```python
from build123d import *

# Parameters (mm, degrees)
D24_5_5_D6_5_2_R                = 12
D24_5_5_D6_5_2_R_2              = 3.25
D24_5_5_D6_5_DEPTH              = 5.5
EXTRUDE_START                   = 5.5
SKETCH_D9_8_1_5_R               = 4.9
SKETCH_D9_8_1_5_R_2             = 3.25
EXTRUDE_D9_8_1_5_DEPTH          = 1.5
F_4XD3_4_D5_8_PCD16_D           = 3.4
F_4XD3_4_D5_8_PCD16_CBORE_D     = 5.8
F_4XD3_4_D5_8_PCD16_CBORE_DEPTH = 3.8
SKETCH_1093_R                   = 10.05
CUT_EXTRUDE_D20_1_0_6_DEPTH     = 0.6
F_4XM2X0_4_PCD14_D              = 1.6


with BuildPart() as part:
    # D24__5.5__D6.5 2 → D24__5.5__D6.5 (new body)
    with BuildSketch(Plane.XY):
        Circle(D24_5_5_D6_5_2_R)
        Circle(D24_5_5_D6_5_2_R_2, mode=Mode.SUBTRACT)
    extrude(amount=D24_5_5_D6_5_DEPTH)

    # 轴承内孔定位台_D9.8_高1.5_截面 → 轴承内孔定位台_D9.8_高1.5 (add)
    with BuildSketch(Plane.XY.offset(EXTRUDE_START)):
        Circle(SKETCH_D9_8_1_5_R)
        Circle(SKETCH_D9_8_1_5_R_2, mode=Mode.SUBTRACT)
    extrude(amount=EXTRUDE_D9_8_1_5_DEPTH)

    # 轴承内圈_4xD3.4通孔_D5.8沉孔_PCD16 (through all)
    with Locations(Plane(origin=(5.656854249, -5.656854249, 0), x_dir=(-1, 0, 0), z_dir=(0, 0, -1))):
        with Locations((0, 0), (11.313708498, 0), (11.313708498, 11.313708498), (0, 11.313708498)):
            CounterBoreHole(F_4XD3_4_D5_8_PCD16_D / 2, F_4XD3_4_D5_8_PCD16_CBORE_D / 2, F_4XD3_4_D5_8_PCD16_CBORE_DEPTH)

    # Sketch 1093 → 原舵盘定位槽_D20.1_深0.6 (cut)
    with BuildSketch(Plane.XY):
        Circle(SKETCH_1093_R)
    extrude(amount=CUT_EXTRUDE_D20_1_0_6_DEPTH, mode=Mode.SUBTRACT)

    # 原舵盘_4xM2x0.4通螺纹_PCD14 (through all)
    with Locations(Plane(origin=(0, -7, 0.6), x_dir=(-1, 0, 0), z_dir=(0, 0, -1))):
        with Locations((0, 0), (7, 7), (0, 14), (-7, 7)):
            Hole(F_4XM2X0_4_PCD14_D / 2)


solid = part.part
```
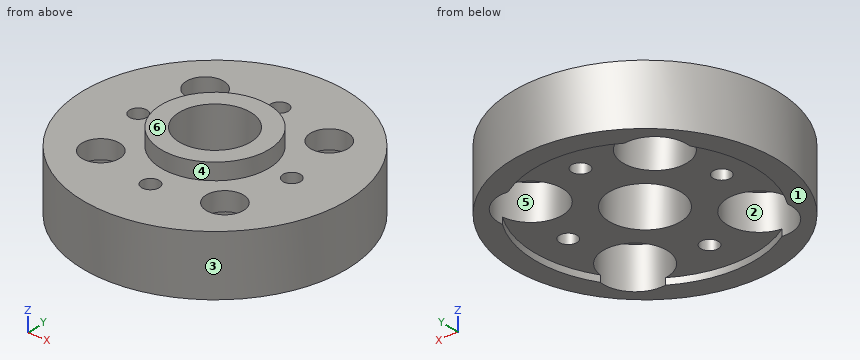
The model under review builds one solid part; all positions refer to its coordinate system, in mm. Face numbers are marked on the shaded views. A direction names the side the tool comes from. Coordinates: 2 decimals unless noted, no trailing zeros. Order: outer loops, then holes, each group sorted by start corner. A loop starts at its lowest first (then second) coordinate and runs counter-clockwise, first axis right, second up. Notation, with made-up numbers: (54, 52) -> (104, 52) arc R26 ccw to (104, 74) -> close; hole circle Ø5 at (83.25, -34). An arc over 180 degrees is marked (long way). Answer in a Markdown table with one row per item. Add a question column.
Item 1: Machinability: for the marked faces 4, 5 and 6, which of the approach directions +Z, -Z, +X, -X, +Y, -Y give a long, thin tool a straight path to every point of the face, cutting with its end or side? Answer none if there is none.
Item 2: We need section B-B on y = -4.5. Write out the cut boundary in (x, z), plus the area to 3 significant figures.
Item 3: To check wall thickness, follow probe 1 along Y at (x, z) = (4, 2.5); probe 2 along X at (y, z) = (-4.5, 5.25); probe 3 along X at (y, z) = (-5.5, 4). State the ranges of each line that lie inside material, in increasing order.
Item 4: Clearance check with flat-ended pins moving along their axes: pin 1 (5.5 mm diameter, centred on x = -5.66, y = 5.66, fed in from +Z); pin 2 (2 mm diameter, centred on y = 5, z = 4.5, fed in from -X); pin 3 (6.5 mm diameter, centred on x = -6.5, y = 6.5, fed in from -Z); pin 4 (2 mm diameter, centred on x = -7, y = 0, fed in from -Z). State where each tip first meets the part, or that it passes through.
Item 5: Mouldability with a two-part tool opening along X and no side actions: class the marked faces 1, 2 and 3 as +X half, -X half, draft (parallel to the pull), parting line (faces both ways), or undercut.
Item 6: We need section A-A on x = 0. Write out the cut boundary in (y, z), plus the area to 3 significant figures.
Item 7: We need section D-D on z = 6.5. Write out the cut boundary in (x, y).
Final values:
| question | item | result |
|---|---|---|
| 1 | face 4 | +Z |
| 1 | face 5 | -Z |
| 1 | face 6 | +Z, +X, -X, +Y, -Y |
| 2 | outline | (-11.12, 0) -> (-8.99, 0) -> (-8.99, 0.6) -> (-8.32, 0.6) -> (-8.32, 3.8) -> (-6.9, 3.8) -> (-6.9, 5.5) -> (-11.12, 5.5) -> close; (-4.41, 3.8) -> (-3, 3.8) -> (-3, 0.6) -> (3, 0.6) -> (3, 3.8) -> (4.41, 3.8) -> (4.41, 5.5) -> (1.94, 5.5) -> (1.94, 7) -> (-1.94, 7) -> (-1.94, 5.5) -> (-4.41, 5.5) -> close; (6.9, 3.8) -> (8.32, 3.8) -> (8.32, 0.6) -> (8.99, 0.6) -> (8.99, 0) -> (11.12, 0) -> (11.12, 5.5) -> (6.9, 5.5) -> close |
| 2 | area | 74.9 mm2 |
| 3 | probe 1 | y = -11.31 to -8.04, -3.28 to 3.28, 8.04 to 11.31 |
| 3 | probe 2 | x = -11.12 to -6.9, -4.41 to 4.41, 6.9 to 11.12 |
| 3 | probe 3 | x = -10.67 to -7.35, -3.96 to 3.96, 7.35 to 10.67 |
| 4 | pin 1 | stops at z = 5.5 |
| 4 | pin 2 | stops at x = -11.31 |
| 4 | pin 3 | stops at z = 0 |
| 4 | pin 4 | stops at z = 0.6 |
| 5 | face 1 | draft |
| 5 | face 2 | undercut |
| 5 | face 3 | parting line |
| 6 | outline | (-12, 0) -> (-10.05, 0) -> (-10.05, 0.6) -> (-7.8, 0.6) -> (-7.8, 5.5) -> (-12, 5.5) -> close; (-6.2, 0.6) -> (-3.25, 0.6) -> (-3.25, 7) -> (-4.9, 7) -> (-4.9, 5.5) -> (-6.2, 5.5) -> close; (3.25, 0.6) -> (6.2, 0.6) -> (6.2, 5.5) -> (4.9, 5.5) -> (4.9, 7) -> (3.25, 7) -> close; (7.8, 0.6) -> (10.05, 0.6) -> (10.05, 0) -> (12, 0) -> (12, 5.5) -> (7.8, 5.5) -> close |
| 6 | area | 77.4 mm2 |
| 7 | outline | circle Ø9.8 at (0, 0); hole circle Ø6.5 at (0, 0) |
